```python
from build123d import *

# Parameters (mm, degrees)
SKETCH1_R                  = 93.345
BASE_DEPTH                 = 4.7625
BASE_DEPTH_BACK            = 4.7625
BOTTOM_SUPPORT_HOLES_DEPTH = 10.525
BOTTOM_SUPPORT_GUIDE_DEPTH = 12.7
SKETCH6_R                  = 1.27
BOTTOM_BOLT_HOLE_DEPTH     = 12.7
TOP_SUPPORT_HOLES_DEPTH    = 4.7625
TOP_SUPPORT_GUIDE_DEPTH    = 12.7
SKETCH12_R                 = 1.27
TOP_BOLT_HOLE_DEPTH        = 12.7
BOTTOM_PATTERN_COUNT       = 4
CIRPATTERN3_COUNT          = 4
SKETCH13_R                 = 19.05
GIMBAL_HOLE_DEPTH          = 25.908


with BuildPart() as part:
    # Sketch1 → Base (new body, two sides)
    with BuildSketch(Plane(origin=(0, 0, 0), x_dir=(1, 0, 0), z_dir=(0, 1, 0))) as base_sk:
        Circle(SKETCH1_R)
    extrude(amount=BASE_DEPTH)
    extrude(base_sk.sketch, amount=-BASE_DEPTH_BACK)

    # Sketch2 → Bottom support holes (cut, through all)
    with BuildSketch(Plane(origin=(0, 4.7625, 0), x_dir=(1, 0, 0), z_dir=(0, 1, 0))):
        with BuildLine():
            Line((0, 88.9), (0, 83.82))
            ThreePointArc((0, 83.82), (-21.72026739, 80.956916842), (-41.956713931, 72.563258996))
            Line((-41.956713931, 72.563258996), (-44.39288973, 77.022602796))
            ThreePointArc((-44.39288973, 77.022602796), (-22.977169228, 85.879332172), (0, 88.9))
        make_face()
    bottom_support_holes = extrude(amount=-BOTTOM_SUPPORT_HOLES_DEPTH, mode=Mode.SUBTRACT)

    # Sketch3 → Bottom support guide (add)
    with BuildSketch(Plane(origin=(0, 4.7625, 0), x_dir=(1, 0, 0), z_dir=(0, 1, 0))):
        with BuildLine():
            Line((0, 83.82), (0, 76.2))
            ThreePointArc((0, 76.2), (-19.834896001, 73.573207764), (-38.302281481, 65.8739344))
            Line((-38.302281481, 65.8739344), (-41.956713931, 72.563258996))
            ThreePointArc((-41.956713931, 72.563258996), (-21.72026739, 80.956916842), (0, 83.82))
        make_face()
    bottom_support_guide = extrude(amount=BOTTOM_SUPPORT_GUIDE_DEPTH)

    # Sketch6 → Bottom bolt hole (cut, symmetric)
    with BuildSketch(Plane(origin=(-20.978356966, 0, -78.191629498), x_dir=(-0.965842482, 0, 0.25912989), z_dir=(-0.25912989, 0, -0.965842482))):
        with Locations((-0.00326739, 11.1125)):
            Circle(SKETCH6_R)
    bottom_bolt_hole = extrude(amount=BOTTOM_BOLT_HOLE_DEPTH, both=True, mode=Mode.SUBTRACT)

    # Sketch8 → Top support holes (cut)
    with BuildSketch(Plane(origin=(-31.122978549, 4.7625, 77.296707326), x_dir=(1, 0, 0), z_dir=(0, 1, 0))):
        with BuildLine():
            Line((-31.738814298, 140.158500173), (-28.14671185, 136.566397725))
            ThreePointArc((-28.14671185, 136.566397725), (-41.480754694, 119.183343848), (-49.854870889, 98.93880289))
            Line((-49.854870889, 98.93880289), (-54.730739557, 100.369398703))
            ThreePointArc((-54.730739557, 100.369398703), (-45.850191767, 121.775253295), (-31.738814298, 140.158500173))
        make_face()
    top_support_holes = extrude(amount=-TOP_SUPPORT_HOLES_DEPTH, mode=Mode.SUBTRACT)

    # Sketch10 → Top support guide (add)
    with BuildSketch(Plane(origin=(-31.122978549, 4.7625, 77.296707326), x_dir=(1, 0, 0), z_dir=(0, 1, 0))):
        with BuildLine():
            Line((-28.14671185, 136.566397725), (-22.758558177, 131.178244052))
            ThreePointArc((-22.758558177, 131.178244052), (-34.92652504, 115.295431983), (-42.540730139, 96.792810073))
            Line((-42.540730139, 96.792810073), (-49.854870889, 98.93880289))
            ThreePointArc((-49.854870889, 98.93880289), (-41.480754694, 119.183343848), (-28.14671185, 136.566397725))
        make_face()
    top_support_guide = extrude(amount=TOP_SUPPORT_GUIDE_DEPTH)

    # Sketch12 → Top bolt hole (cut, symmetric)
    with BuildSketch(Plane(origin=(-70.123769919, 0, -40.455892982), x_dir=(-0.499721266, 0, 0.866186271), z_dir=(-0.866186271, 0, -0.499721266))):
        with Locations((-0.00326739, 11.1125)):
            Circle(SKETCH12_R)
    top_bolt_hole = extrude(amount=TOP_BOLT_HOLE_DEPTH, both=True, mode=Mode.SUBTRACT)

    # Bottom pattern: Bottom support holes, Bottom support guide, Bottom bolt hole ×4 about axis
    bottom_pattern_axis = Axis((0, 0, 0), (0, 1, 0))
    for i in range(1, BOTTOM_PATTERN_COUNT):
        add(bottom_support_holes.rotate(bottom_pattern_axis, i * 360 / BOTTOM_PATTERN_COUNT), mode=Mode.SUBTRACT)
        add(bottom_support_guide.rotate(bottom_pattern_axis, i * 360 / BOTTOM_PATTERN_COUNT))
        add(bottom_bolt_hole.rotate(bottom_pattern_axis, i * 360 / BOTTOM_PATTERN_COUNT), mode=Mode.SUBTRACT)

    # CirPattern3: Top support holes, Top support guide, Top bolt hole ×4 about axis
    cirpattern3_axis = Axis((0, 0, 0), (0, 1, 0))
    for i in range(1, CIRPATTERN3_COUNT):
        add(top_support_holes.rotate(cirpattern3_axis, i * 360 / CIRPATTERN3_COUNT), mode=Mode.SUBTRACT)
        add(top_support_guide.rotate(cirpattern3_axis, i * 360 / CIRPATTERN3_COUNT))
        add(top_bolt_hole.rotate(cirpattern3_axis, i * 360 / CIRPATTERN3_COUNT), mode=Mode.SUBTRACT)

    # Sketch13 → Gimbal Hole (cut)
    with BuildSketch(Plane(origin=(0, 4.7625, 0), x_dir=(1, 0, 0), z_dir=(0, 1, 0))):
        Circle(SKETCH13_R)
    extrude(amount=-GIMBAL_HOLE_DEPTH, mode=Mode.SUBTRACT)


solid = part.part
```
Geometry check sheet. Reference: the model listing, model coordinates, mm. A direction names the side the tool comes from. Round coordinates to 2 decimals unless told otherwise and drop trailing zeros. Loops run counter-clockwise (first coordinate to the right, second up) from the corner with the lowest first, then second, coordinate; pieces in that order, holes last. Notation, with made-up numbers: (6, 33) -> (19, 33) arc R21 cw to (19, 53) -> close; hole circle Ø1 at (30, 53). An arc over 180 degrees is marked (long way). Use a Markdown table: item, result.
(1) Go/stop test with flat-tipped pins: P1, Ø6, axis at x = -78.5, y = 9.5, coming from the -Z side; P2, Ø4, axis at y = -1.5, z = 86.5, coming from the +X side; P3, Ø2.5, axis at x = 86.5, y = -2, coming from the -Z side. Record where each tip stops, or that it passes through.
Calculated:
| item | result |
|---|---|
| P1 | z = -36.41 |
| P2 | x = 39.66 |
| P3 | z = -38.02 |
(2) Sectioned sample at A-A (z = -11). Enter the section's corners in (x, y), then the cut area to 3 significant figures.
Calculated:
| item | result |
|---|---|
| outline | (-92.69, -4.76) -> (-15.55, -4.76) -> (-15.55, 4.76) -> (-92.69, 4.76) -> close; (15.55, -4.76) -> (83.1, -4.76) -> (83.1, 17.46) -> (75.4, 17.46) -> (75.4, 4.76) -> (15.55, 4.76) -> close; (88.22, -4.76) -> (92.69, -4.76) -> (92.69, 4.76) -> (88.22, 4.76) -> close |
| area | 1,520 mm² |
(3) Mould release check, pull along Y, two halves, no side actions. Record for faces 6 (the flat face through (43.158, 0.067, 74.762)), 7 (the flat face through (-21, 17.462, -77)), 8 (the cylindrical face through (77.59, 10.34, -19.77)): released by +Y, released by -Y, zero draft, split by the parting line, or undercut.
Calculated:
| item | result |
|---|---|
| face 6 | zero draft |
| face 7 | released by +Y |
| face 8 | undercut |
(4) Sectioned sample at B-B (x = -12). Enter the section's corners in (y, z).
Calculated:
| item | result |
|---|---|
| outline | (-4.76, -92.57) -> (4.76, -92.57) -> (4.76, -88.09) -> (-4.76, -88.09) -> close; (-4.76, -82.96) -> (17.46, -82.96) -> (17.46, -75.25) -> (4.76, -75.25) -> (4.76, -14.8) -> (-4.76, -14.8) -> close; (-4.76, 14.8) -> (4.76, 14.8) -> (4.76, 92.57) -> (-4.76, 92.57) -> close |
(5) Set-up check for faces 1 (the flat face through (74.762, 0.067, -43.158)), 2 (the flat face through (77.27, 11.024, 20.554)), 3 (the cylindrical face through (41.62, 8.609, -72.757)), 4 (the flat face through (68, 17.462, 41)), 5 (the flat face through (0, 11, -80)): record each of +Z, -Z, +X, -X, +Y, -Y from which the full face is reachable in a straight line by a thin tool's end or side.
Calculated:
| item | result |
|---|---|
| face 1 | +Y, -Y |
| face 2 | +X, +Y |
| face 3 | +Y |
| face 4 | +Z, -Z, +X, -X, +Y |
| face 5 | -Z, +Y |
(6) Scan lines: probe 1 along Z at (x, y) = (30, 1.5); probe 2 along Y at (x, z) = (54.5, 41); probe 3 along Z at (x, y) = (58, 7.75). Record each from-to range of solid material in increasing order.
Calculated:
| item | result |
|---|---|
| probe 1 | -88.39 to -83.69, -78.27 to 78.27, 83.69 to 88.39 |
| probe 2 | -4.76 to 4.76 |
| probe 3 | -60.51 to -58, 49.42 to 58 |
